Could you check a few things on this model? Use its own coordinates, in mm. A direction names the side the tool comes from. Coordinates: 2 decimals unless noted, no trailing zeros. Order: outer loops, then holes, each group sorted by start corner. A loop starts at its lowest first (then second) coordinate and runs counter-clockwise, first axis right, second up. Notation, with made-up numbers: (-6, -14) -> (28, -14) arc R24 cw to (28, -1) -> close; hole circle Ø6 at (80, 7). An arc over 180 degrees is marked (long way). Return JSON: item names as keys, results as strings. Group by question number.
from build123d import *

# Parameters (mm, degrees)
SKETCH_R        = 2.25
SKETCH_R_2      = 11.25
SKETCH_R_3      = 1.75
PAD_DEPTH       = 23
POCKET_DEPTH    = 19
SKETCH004_R     = 2.25
POCKET003_DEPTH = 10
SKETCH005_R     = 4.05
POCKET004_DEPTH = 12
SKETCH006_R     = 3.75
POCKET005_DEPTH = 10


with BuildPart() as pocket005:
    # Sketch → Pad (new body)
    with BuildSketch(Plane.XY):
        Polygon((0, 0), (105, 0), (105, 62), (20, 62), (20, 42), (0, 42), align=None)
        with Locations((38, 10)):
            Circle(SKETCH_R, mode=Mode.SUBTRACT)
        with Locations((33, 35)):
            Circle(SKETCH_R, mode=Mode.SUBTRACT)
        with Locations((84, 21)):
            Circle(SKETCH_R_2, mode=Mode.SUBTRACT)
        with Locations((68.5, 36.5)):
            Circle(SKETCH_R_3, mode=Mode.SUBTRACT)
        with Locations((99.5, 36.5)):
            Circle(SKETCH_R_3, mode=Mode.SUBTRACT)
        with Locations((68.5, 5.5)):
            Circle(SKETCH_R_3, mode=Mode.SUBTRACT)
        with Locations((99.5, 5.5)):
            Circle(SKETCH_R_3, mode=Mode.SUBTRACT)
        with Locations((10, 30)):
            Circle(SKETCH_R, mode=Mode.SUBTRACT)
        with Locations((10, 15)):
            Circle(SKETCH_R, mode=Mode.SUBTRACT)
        with Locations((42, 52)):
            Circle(SKETCH_R, mode=Mode.SUBTRACT)
        with Locations((94, 52)):
            Circle(SKETCH_R, mode=Mode.SUBTRACT)
        with BuildLine():
            Line((58.75, 25), (58.75, 39.999999))
            ThreePointArc((58.75, 39.999999), (56.5, 42.25), (54.25, 39.999998))
            Line((54.25, 25.000001), (54.25, 39.999998))
            ThreePointArc((54.25, 25.000001), (56.5, 22.75), (58.75, 25))
        make_face(mode=Mode.SUBTRACT)
    extrude(amount=PAD_DEPTH)

    # Sketch001 → Pocket (cut)
    with BuildSketch(Plane.XY.offset(23)):
        with BuildLine():
            ThreePointArc((41.485277, 42), (39.015593, 44.209375), (35.999996, 45.583005))
            Line((35.999996, 67), (35.999996, 45.583005))
            Line((20, 67), (35.999996, 67))
            Line((20, -1), (20, 67))
            Line((20, -1), (48.252269, -1))
            Line((48.252269, 11), (48.252269, -1))
            Line((48.252269, 11), (70.252269, 11))
            ThreePointArc((70.252269, 11), (71.759618, 9.202833), (73.499996, 7.630258))
            Line((73.499996, 7.630258), (73.499996, -1))
            Line((73.499996, -1), (93.499996, -1))
            Line((93.499996, -1), (93.499996, 6.902128))
            ThreePointArc((93.499996, 6.902128), (95.574295, 8.548671), (97.367695, 10.497399))
            Line((105.499996, 10.497399), (97.367695, 10.497399))
            Line((105.499996, 30.497399), (105.499996, 10.497399))
            Line((98.099621, 30.497399), (105.499996, 30.497399))
            ThreePointArc((98.099621, 30.497399), (91.98574, 36.007594), (83.999996, 38))
            Line((83.999996, 38), (83.999996, 67))
            Line((83.999996, 67), (46.999996, 67))
            Line((46.999996, 67), (46.999996, 42))
            Line((41.485277, 42), (46.999996, 42))
        make_face()
    extrude(amount=-POCKET_DEPTH, mode=Mode.SUBTRACT)

    # Sketch004 → Pocket003 (cut)
    with BuildSketch(Plane.XY.offset(23)):
        with Locations((55, 5)):
            Circle(SKETCH004_R)
    extrude(amount=-POCKET003_DEPTH, mode=Mode.SUBTRACT)

    # Sketch005 → Pocket004 (cut)
    with BuildSketch(Plane.XZ):
        with Locations((13, 16)):
            Circle(SKETCH005_R)
    extrude(amount=-POCKET004_DEPTH, mode=Mode.SUBTRACT)

    # Sketch006 → Pocket005 (cut)
    with BuildSketch(Plane(origin=(0, 0, 0), x_dir=(1, 0, 0), z_dir=(0, 0, -1))):
        with Locations((10, -15)):
            Circle(SKETCH006_R)
        with Locations((10, -30)):
            Circle(SKETCH006_R)
        with Locations((42, -52)):
            Circle(SKETCH006_R)
        with Locations((94, -52)):
            Circle(SKETCH006_R)
    extrude(amount=-POCKET005_DEPTH, mode=Mode.SUBTRACT)


with BuildPart() as part_mirroring:
    # Part__Mirroring: instance of Pocket005
    add(pocket005.part.mirror(Plane(origin=(0, 0, 0), x_dir=(0, -1, 0), z_dir=(1, 0, 0))))


solid = part_mirroring.part
Q1. I'm going to push flat-ended pins straight in: pin 1 Ø2 at (x, y) = (-94, 52.5) entering from -Z; pin 2 Ø2 at (y, z) = (47.5, 2.5) entering from +X; pin 3 Ø1.7 at (x, z) = (-43.5, 13.5) entering from -Y; pin 4 Ø7 at (x, y) = (-42, 52) entering from -Z. Where does each tip first touch, or does it pass through?
Q2. I want a section at B-B on y = 21. Please give me the cut outline in (x, z).
Q3. On a 3-axis mill with a long thin cutter (end or side, diameter ignored), from which of +Z, -Z, +X, -X, +Y, -Y can I reach the whole of each face in a straight line? I mean faces 4 (the flat face through (-93.5, 3, 14)), 5 (the flat face through (-54.25, 32, 2)), 6 (the flat face through (-96, 54, 10)), 7 (the flat face through (-101, 10.497, 14)). Say none if no direction works.
Q4. We'd pull the mould along X, two halves only. Please class faces 1 (the flat face through (-52, 0, 9)), 2 (the cylindrical face through (-95.547, 8.523, 13.633)), 3 (the flat face through (-20, 52, 2)): pulls with the +X half, pulls with the -X half, needs draft (parallel to the pull), parting line crosses it, or undercut.
Q5. I want a section at A-A on x = -99.5. Please give me the cut outline in (y, z).
Q6. I want a section at D-D on z = 14.25. State how many separate pieces and enclosed holes the cut face has, and give its area (3 significant figures).
Q7. I want a section at C-C on x = -88.5. Please give me the cut outline in (y, z).
Q8. I need wall thicknesses on line 1 along Y through (x, z) = (-94, 4.5); line 2 along Y through (x, z) = (-10, 20); line 3 along X through (y, z) = (15, 7.75). Which ranges of each line are inside material? Lowest first, please. Write a range as from..to.
Response values:
{
 "1": {"pin 1": "passes through", "pin 2": "stops at x = -20", "pin 3": "stops at y = 42", "pin 4": "stops at z = 10"},
 "2": {"outline": "(-105, 0) -> (-95.25, 0) -> (-95.25, 4) -> (-105, 4) -> close; (-72.75, 0) -> (0, 0) -> (0, 23) -> (-20, 23) -> (-20, 4) -> (-72.75, 4) -> close"},
 "3": {"face 4": "+Z, -Y", "face 5": "+Z, -Z", "face 6": "-Z", "face 7": "+Z, -X"},
 "4": {"face 1": "needs draft", "face 2": "undercut", "face 3": "pulls with the +X half"},
 "5": {"outline": "(0, 0) -> (3.75, 0) -> (3.75, 23) -> (0, 23) -> close; (7.25, 0) -> (34.75, 0) -> (34.75, 23) -> (30.5, 23) -> (30.5, 4) -> (10.5, 4) -> (10.5, 23) -> (7.25, 23) -> close; (38.25, 0) -> (62, 0) -> (62, 23) -> (38.25, 23) -> close"},
 "6": {"separate pieces": "5", "enclosed holes": "8", "area": "1,820 mm²"},
 "7": {"outline": "(0, 0) -> (10.69, 0) -> (10.69, 4) -> (0, 4) -> close; (31.31, 0) -> (62, 0) -> (62, 23) -> (37.39, 23) -> (37.39, 4) -> (31.31, 4) -> close"},
 "8": {"line 1": "y = 0..7.25, 34.75..48.25, 55.75..62", "line 2": "y = 0..12.75, 17.25..27.75, 32.25..42", "line 3": "x = -20..-13.75, -6.25..0"}
}
